Can you work these out from the model? Positions are in its coordinate system, mm. Face numbers are marked on the shaded views. A direction names the side the tool comes from. Coordinates: 2 decimals unless noted, no trailing zeros. Order: outer loops, then holes, each group sorted by start corner. A loop starts at its lowest first (then second) coordinate and runs counter-clockwise, first axis right, second up. Notation, with made-up numbers: (89, 47.25) -> (142, 47.25) arc R4 cw to (142, 52.25) -> close; hole circle Ø11 at (48, 80). An arc over 180 degrees is marked (long way). Answer as a JSON object with one key per item and string values. Group by question number.
(1) I want a section at A-A, the plane x = 0. List the corners of the cut face in (y, z) for me (3 decimals), plus the area to 3 significant figures.
(2) I need wall thicknesses on line 1 (Z direction, x = 0, y = 0.5); line 2 (Z direction, x = 0, y = 6.5) (1 decimal); line 3 (Y direction, x = -3.25, z = 0.5). Which ranges of each line are inside material? Lowest first, please.
(3) If we mould it in two halves opening along X, with no side actions, what happens to the marked faces 3, 4 and 5? For each: pulls with the +X half, pulls with the -X half, needs draft (parallel to the pull), parting line crosses it, or undercut.
(4) I want a section at C-C, the plane y = 10.75. List the corners of the cut face in (x, z) for me (3 decimals), plus the area to 3 significant figures.
(5) I want a section at B-B, the plane z = 0. List the corners of the cut face in (x, y) for me (3 decimals), plus the area to 3 significant figures.
(6) For pin 1 (5 mm diameter, centred on x = -4, y = 12.5, fed in from -Z); pin 2 (3 mm diameter, centred on x = 4.5, z = -1, fed in from -Y); pin 3 (3 mm diameter, centred on x = -1, y = 11.5, fed in from +Z); pin 4 (1 mm diameter, centred on x = 4.5, y = 6, fed in from +Z), each with a flat end and sliding along its axis, tell me the tip position at first contact or that it passes through.
(7) I want a section at D-D, the plane y = 1.75. List the corners of the cut face in (x, z) for me.
(8) Which directions (+Z, -Z, +X, -X, +Y, -Y) give clear straight access to the entire face, cutting with the end or side of a thin tool? Please do the marked faces 1 and 2.
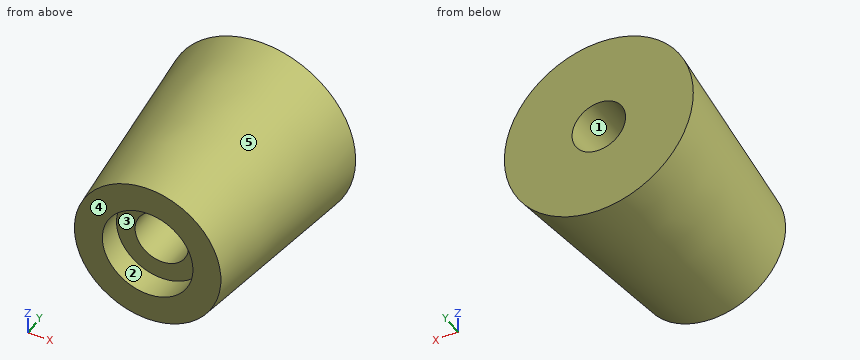
Autodesk Inventor part; units mm, degrees
ref_plane "YZ Plane" through (0, 0, 0) normal (1, 0, 0) x (0, 1, 0)
ref_plane "XZ Plane" through (0, 0, 0) normal (0, 1, 0) x (-1, 0, 0)
ref_plane "XY Plane" through (0, 0, 0) normal (0, 0, 1) x (1, 0, 0)
sketch "Esquisse3" plane through (0, 0, 0) normal (0, 1, 0) x (-1, 0, 0)
  circle A0 centre (0, 0) radius 2.125
  circle A1 centre (0, 0) radius 7.5
  dimension "d12" = 4.25
  dimension "d13" = 15
extrude "Extrusion3" add sketch "Esquisse3" along normal blind 16
draft "Dépouille de face1" angle 6 pull direction (0, -1, 0) faces at (-7.4757, 10.6667, -0.6035) fixed edges at (7.5, 16, 0)
sketch "Esquisse4" plane through (0, 16, 0) normal (0, 1, 0) x (1, 0, 0)
  point P0 (0, 0)
sketch "Esquisse6" plane through (0, 0, 0) normal (0, -1, 0) x (1, 0, 0)
  circle A0 centre (0, 0) radius 3.6
  dimension "d22" = 7.2
extrude "Extrusion5" cut sketch "Esquisse6" against normal blind 2
properties part number "cleat"
Computed values:
{
 "1": {"outline": "(0, -5.818) -> (16, -7.5) -> (16, -2.125) -> (2, -2.125) -> (2, -3.6) -> (0, -3.6) -> close; (0, 3.6) -> (2, 3.6) -> (2, 2.125) -> (16, 2.125) -> (16, 7.5) -> (0, 5.818) -> close", "area": "139 mm2"},
 "2": {"line 1": "z = -5.87 to -3.6, 3.6 to 5.87", "line 2": "z = -6.5 to -2.1, 2.1 to 6.5", "line 3": "y = 2 to 16"},
 "3": {"face 3": "undercut", "face 4": "needs draft", "face 5": "parting line crosses it"},
 "4": {"outline": "circle Ø13.896 at (0, 0); hole circle Ø4.25 at (0, 0)", "area": "137 mm2"},
 "5": {"outline": "(-7.5, 16) -> (-5.818, 0) -> (-3.6, 0) -> (-3.6, 2) -> (-2.125, 2) -> (-2.125, 16) -> close; (2.125, 2) -> (3.6, 2) -> (3.6, 0) -> (5.818, 0) -> (7.5, 16) -> (2.125, 16) -> close", "area": "139 mm2"},
 "6": {"pin 1": "stops at z = -7.03", "pin 2": "stops at y = 0", "pin 3": "stops at z = 7.16", "pin 4": "stops at z = 5.06"},
 "7": {"outline": "circle Ø12 at (0, 0); hole circle Ø7.2 at (0, 0)"},
 "8": {"face 1": "+Y, -Y", "face 2": "-Y"}
}
